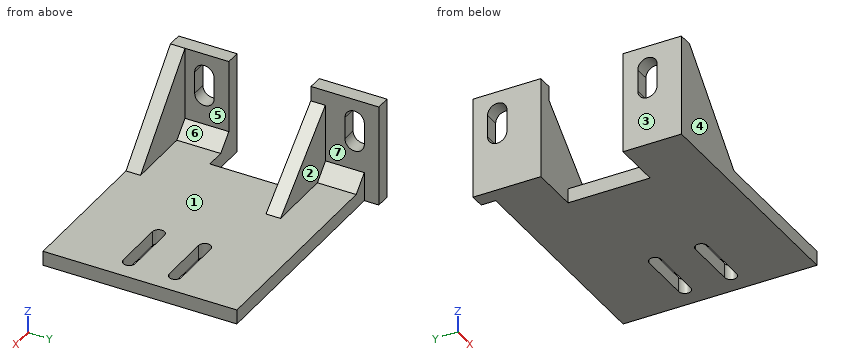
Autodesk Inventor part; units mm, degrees
ref_plane "YZ Plane" through (0, 0, 0) normal (1, 0, 0) x (0, 1, 0)
ref_plane "XZ Plane" through (0, 0, 0) normal (0, 1, 0) x (-1, 0, 0)
ref_plane "XY Plane" through (0, 0, 0) normal (0, 0, 1) x (1, 0, 0)
sketch "Sketch1" plane through (0, 0, 0) normal (0, 0, 1) x (1, 0, 0)
  line L0 (0, 0) -> (50, 0)
  line L1 (50, 0) -> (50, -40)
  line L2 (50, -40) -> (0, -40)
  line L3 (0, -40) -> (0, 0)
  dimension "d0" = 50
  dimension "d1" = 40
extrude "Extrusion1" add sketch "Sketch1" along normal blind 3
sketch "Sketch2" plane through (0, 0, 3) normal (0, 0, 1) x (1, 0, 0)
  line L0 (0, -40) -> (50, -40)
  line L1 (0, 0) -> (3, 0)
  line L2 (3, 0) -> (3, -40)
  line L3 (3, -40) -> (0, -40)
  line L4 (0, -40) -> (0, 0)
  dimension "d4" = 3
extrude "Extrusion2" add sketch "Sketch2" along normal blind 18
sketch "Sketch3" plane through (0, 0, 0) normal (0, 1, 0) x (1, 0, 0)
  line L0 (0, 0) -> (3, 0)
  line L1 (3, 0) -> (3, -21)
  line L2 (3, -21) -> (0, -21)
  line L3 (0, -21) -> (0, 0)
extrude "Extrusion3" add sketch "Sketch3" along normal blind 3
sketch "Sketch4" plane through (0, 0, 0) normal (0, 0, -1) x (-1, 0, 0)
  line L0 (0, -40) -> (0, 3)
  line L1 (-3, 0) -> (-3, 3)
  line L2 (-3, 0) -> (-3, -11)
  line L3 (0, -11) -> (-10, -11)
  line L4 (-10, -11) -> (-10, -27.9486)
  line L5 (-10, -27.9486) -> (0, -27.9486)
  point P0 (0, 0)
  dimension "d9" = 11
  dimension "d10" = 10
extrude "Extrusion4" cut sketch "Sketch4" against normal blind 8
sketch "Sketch6" plane through (0, -40, 0) normal (-1, 0, 0) x (0, 0, 1)
  line L0 (0, 29) -> (8, 29)
  line L1 (12, 38) -> (16.5475, 38) construction
  line L2 (12, 36) -> (16.5475, 36)
  line L3 (16.5475, 40) -> (12, 40)
  arc A0 (12, 40) -> (12, 36) centre (12, 38) ccw
  arc A1 (16.5475, 36) -> (16.5475, 40) centre (16.5475, 38) ccw
  point P0 (0, 40)
  point P1 (14.2738, 38)
extrude "Extrusion6" cut sketch "Sketch6" against normal through all
sketch "Sketch7" plane through (0, -40, 0) normal (-1, 0, 0) x (0, 0, 1)
  line L0 (16.5475, 36) -> (12, 36)
  line L1 (12, 7) -> (16.5475, 7) construction
  line L2 (12, 5) -> (16.5475, 5)
  line L3 (16.5475, 9) -> (12, 9)
  arc A0 (12, 9) -> (12, 5) centre (12, 7) ccw
  arc A1 (16.5475, 5) -> (16.5475, 9) centre (16.5475, 7) ccw
  point P0 (0, 40)
  point P1 (14.2738, 7)
  dimension "d67" = 4
extrude "Extrusion7" cut sketch "Sketch7" against normal through all
sketch "Sketch8" plane through (0, 0, 0) normal (0, 0, -1) x (-1, 0, 0)
  line L0 (0, -27.9486) -> (-10, -27.9486)
  line L1 (-57.8737, -20) -> (-13.9473, -20) construction
  line L2 (-46.7188, -20) -> (-46.7188, -15.25) construction
  line L3 (-46.7188, -15.25) -> (-19.9847, -15.25) construction
  line L4 (-19.9847, -15.25) -> (-19.9847, -24.75) construction
  line L5 (-19.9847, -24.75) -> (-61.1977, -24.75) construction
  line L6 (-46.7188, -15.25) -> (-33.3518, -15.25) construction
  line L7 (-45.4688, -16.5) -> (-34.6018, -16.5)
  line L8 (-34.6018, -14) -> (-45.4688, -14)
  arc A0 (-45.4688, -14) -> (-45.4688, -16.5) centre (-45.4688, -15.25) ccw
  arc A1 (-34.6018, -16.5) -> (-34.6018, -14) centre (-34.6018, -15.25) ccw
  line L9 (-46.7188, -20) -> (-46.7188, -24.9647) construction
  arc A2 (-33.3518, -15.25) -> (-33.4221, -15.7265) centre (-33.3518, -15.4935) ccw construction
  line L10 (-33.4221, -15.7265) -> (-33.4221, -27.1874) construction
  line L11 (-46.7188, -24.75) -> (-33.4221, -24.75) construction
  line L12 (-45.4688, -26) -> (-34.6721, -26)
  line L13 (-34.6721, -23.5) -> (-45.4688, -23.5)
  arc A3 (-45.4688, -23.5) -> (-45.4688, -26) centre (-45.4688, -24.75) ccw
  arc A4 (-34.6721, -26) -> (-34.6721, -23.5) centre (-34.6721, -24.75) ccw
  point P0 (0, 0)
  point P1 (-40.0353, -15.25)
  point P2 (-40.0705, -24.75)
  dimension "d71" = 4.75
  dimension "d72" = 9.5
  dimension "d73" = 2.5
  dimension "d76" = 2.5
chamfer "Chamfer1" distance 3 angle 45 1 edges at (3, -33.9743, 3)
chamfer "Chamfer2" distance 3 angle 45 1 edges at (3, -5.5, 3)
sketch "Sketch11" plane through (0, 0, 0) normal (0, 0, -1) x (-1, 0, 0)
  line L0 (-48.6932, -22.9665) -> (-25.0226, -22.9665) construction
  line L1 (-45, -22.9665) -> (-37, -22.9665) construction
  line L2 (-10, -11) -> (0, -11)
  line L3 (0, -11) -> (0, 3)
  line L4 (-3, 3) -> (0, 3)
  line L5 (-3, 0) -> (-3, 3)
  line L6 (-3, 0) -> (-50, 0)
  line L7 (-50, 0) -> (-50, -40)
  line L8 (-50, -40) -> (0, -40)
  line L9 (0, -40) -> (0, -27.9486)
  line L10 (0, -27.9486) -> (-10, -27.9486)
  line L11 (-10, -27.9486) -> (-10, -11)
  point P0 (0, 0)
  point P1 (-41, -22.9665)
ref_plane "Work Plane1" through (0, -8, 0) normal (0, 1, 0) x (1, 0, 0)
sketch "Sketch14" plane through (0, -8, 0) normal (0, 1, 0) x (1, 0, 0)
  line L0 (3.0794, -17.957) -> (19.7008, -2.8939)
  line L1 (19.7008, -2.8939) -> (3.0794, -2.8939)
  line L2 (3.0794, -2.8939) -> (3.0794, -17.957)
  point P0 (0, 0)
extrude "Extrusion14" add sketch "Sketch14" against normal blind 3
sketch "Sketch15" plane through (0, -40, 21) normal (0, -1, 0) x (1, 0, 0)
  line L0 (6, -18) -> (50, -18)
  line L1 (3, -15) -> (6, -18)
  line L2 (3, -15) -> (3, 0)
  line L3 (3, 0) -> (19.3977, -18)
  line L4 (3, -15.75) -> (3, 0)
extrude "Extrusion15" add sketch "Sketch15" against normal blind 3
sketch "Sketch16" plane through (3, 0, 0) normal (1, 0, 0) x (0, 0, -1)
  line L0 (-21, -37) -> (-21, 3)
  line L1 (-21, -11) -> (-8, -11)
  line L2 (-8, -11) -> (-8, -27.9486)
  line L3 (-8, -27.9486) -> (-21, -27.9486)
  line L4 (-21, -27.9486) -> (-21, -11)
extrude "Extrusion16" cut sketch "Sketch16" against normal through all
extrude "Extrusion17" cut sketch "Sketch8" against normal through all contours A0 L8 A1 L7
extrude "Extrusion18" cut sketch "Sketch8" against normal through all contours A3 L13 A4 L12
properties part number "bart z endstop bracket plain switch v1"
Here's how the part is built. I have some questions about the finished solid (model axes, mm). Face numbers are marked on the shaded views. A direction names the side the tool comes from. Coordinates: 2 decimals unless noted, no trailing zeros. Write each loop counter-clockwise with the first axis right and the second up, starting at its lowest first coordinate (ties: lowest second). Pieces come first, ordered by that corner, then holes. Notation, with made-up numbers: M 53,27 L 57,27 A12 cw 57,49 Z; hole C 68.5,10.5 d10. An arc over 180 degrees is marked long. Answer as CSV lines item,"result". Start each with the question number.
Q1. I need wall thicknesses on probe 1 along Y at (x, z) = (4.5, 9.25); probe 2 along Y at (x, z) = (7, 2.25); probe 3 along Z at (x, y) = (39, -35). Which ranges of each line are inside material? Lowest first, please. Write a range as [from, to].
Q2. Suppose I cut it at C-C, the plane z = 13.75. List the corners of the cut face in (x, y) for me.
Q3. For the marked faces 4, 5, 6 and 7, which set-ups out of +Z, -Z, +X, -X, +Y, -Y let a thin tool reach every point of the face, with its end or its side?
Q4. Suppose I cut it at A-A, the plane y = -33. List the corners of the cut face in (x, z) for me.
Q5. Will these pins go through, and if not, where does the flat tip stop? pin 1 Ø5 at (x, z) = (38, 3.5) entering from +Y; pin 2 Ø3.5 at (y, z) = (-19, 1.5) entering from -X; pin 3 Ø1 at (x, y) = (8, -31.5) entering from +Z.
Q6. Suppose I cut it at D-D, the plane y = -24.75. List the corners of the cut face in (x, z) for me, then the cut area to 3 significant figures.
Q7. If we mould it in two halves opening along Y, with no side actions, what happens to the marked faces 1, 2 and 3? For each: pulls with the +Y half, pulls with the -Y half, needs draft (parallel to the pull), parting line crosses it, or undercut.
Q8. Suppose I cut it at B-B, the plane z = 2. List the corners of the cut face in (x, y) for me, then the cut area to 3 significant figures.
Entries:
1,probe 1,"y = [-40, -37], [-11, -8]"
1,probe 2,"y = [-40, -27.95], [-11, 0]"
1,probe 3,"z = [0, 3]"
2,outline,"M 0,-40 L 9.6,-40 L 9.6,-37 L 3,-37 L 3,-35 L 0,-35 Z; M 0,-31 L 3,-31 L 3,-27.95 L 0,-27.95 Z; M 0,-11 L 3,-11 L 3,-4 L 0,-4 Z; M 0,0 L 3,0 L 3,3 L 0,3 Z; M 3.08,-11 L 7.72,-11 L 7.72,-8 L 3.08,-8 Z"
3,face 4,"+Z, -Z, +X, -X, -Y"
3,face 5,"+Z, +X, +Y"
3,face 6,"+Z, +X"
3,face 7,"+Z, +Y"
4,outline,"M 0,0 L 50,0 L 50,3 L 6,3 L 3,6 L 3,10 L 0,10 Z; M 0,18.55 L 3,18.55 L 3,21 L 0,21 Z"
5,pin 1,"stops at y = 0"
5,pin 2,"stops at x = 10"
5,pin 3,"stops at z = 3"
6,outline,"M 10,0 L 33.42,0 L 33.42,3 L 10,3 Z; M 46.72,0 L 50,0 L 50,3 L 46.72,3 Z"
6,area,"80.1 mm²"
7,face 1,"undercut"
7,face 2,"pulls with the +Y half"
7,face 3,"needs draft"
8,outline,"M 0,-40 L 50,-40 L 50,0 L 3,0 L 3,3 L 0,3 L 0,-11 L 10,-11 L 10,-27.95 L 0,-27.95 Z; hole M 34.6,-16.5 L 45.47,-16.5 A1.25 ccw 45.47,-14 L 34.6,-14 A1.25 ccw Z; hole M 34.67,-26 L 45.47,-26 A1.25 ccw 45.47,-23.5 L 34.67,-23.5 A1.25 ccw Z"
8,area,"1,780 mm²"
